The figure shows three views and two pictorial views of one solid part (mm, origin at its lowest corner). Answer the questions. A direction names the side the tool comes from. Coordinates: 2 decimals unless noted, no trailing zeros. Write each loop counter-clockwise with the first axis right and the second up, starting at its lowest first coordinate (ties: lowest second). Pieces come first, ordered by that corner, then holes. Notation, with made-up numbers: M 24.5,25 L 68.5,25 A20 cw 68.5,50 Z; hole C -3.5,86.25 d4. An arc over 180 degrees is marked long. Answer as CSV lines item,"result".
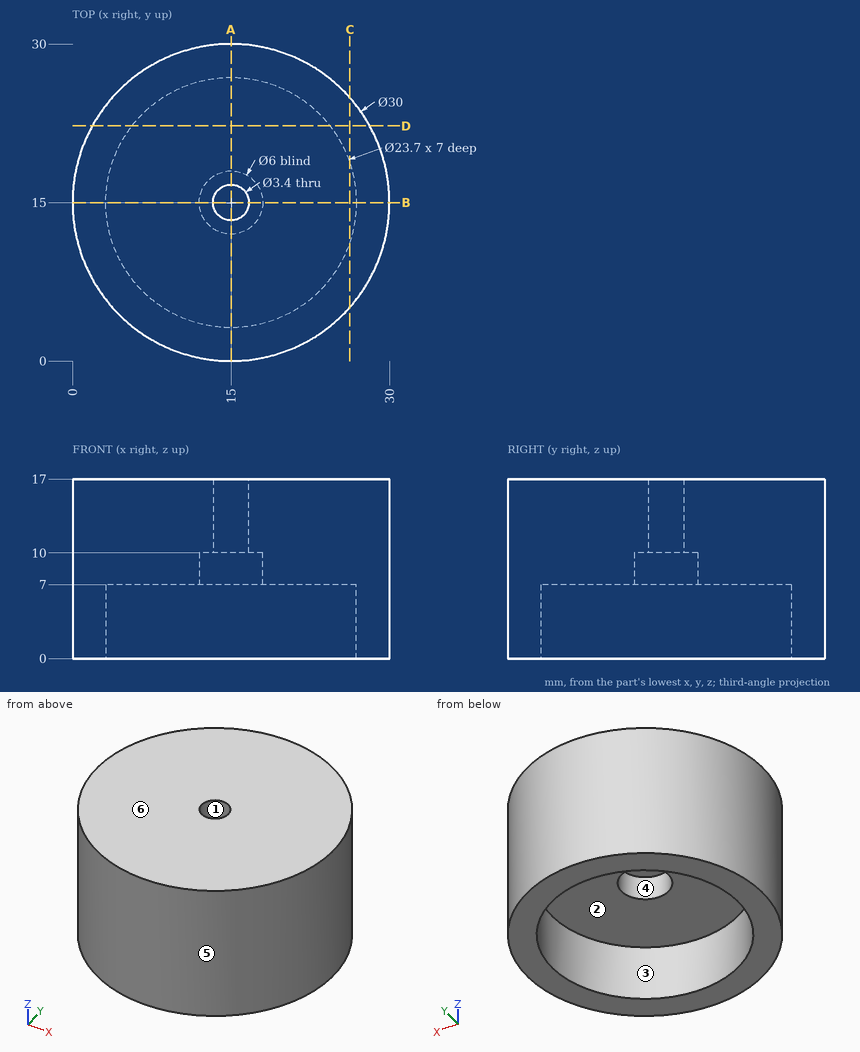
Q1. Flat-ended cylindrical pins translate along their axes: pin 1 Ø7 at (x, y) = (10.5, 20) entering from -Z; pin 2 Ø3 at (x, z) = (8.5, 11.5) entering from -Y; pin 3 Ø4 at (y, z) = (5.5, 6) entering from +X. Find the tip coordinate at first contact, or state that the pin passes through.
Output:
pin 1,"z = 7"
pin 2,"y = 0.86"
pin 3,"x = 27.99"
Q2. Find section D-D (y = 22.25). Give the vertices of the cut face in (x, z), and give its area (3 significant figures).
Output:
outline,"M 1.87,0 L 5.63,0 L 5.63,7 L 24.37,7 L 24.37,0 L 28.13,0 L 28.13,17 L 1.87,17 Z"
area,"315 mm2"
Q3. For the marked faces 1 and 2, determine the directions among +Z, -Z, +X, -X, +Y, -Y from which every point of the face is accessible in a straight line to the end or side of a thin tool.
Output:
face 1,"+Z, -Z"
face 2,"-Z"
Q4. Straight lines are drawn through the part: line 1 (Y direction, x = 15, z = 1.75); line 2 (Y direction, x = 15, z = 8.25); line 3 (Z direction, x = 12.75, y = 26.25). For each, find the intervals that lie inside material, in ascending order.
Output:
line 1,"0 to 3.15, 26.85 to 30"
line 2,"0 to 12, 18 to 30"
line 3,"7 to 17"
Q5. The mould has two halves that part along X. Classify the marked faces 3, 4, 5 and 6: pulls with the +X half, pulls with the -X half, needs draft (parallel to the pull), parting line crosses it, or undercut.
Output:
face 3,"undercut"
face 4,"undercut"
face 5,"parting line crosses it"
face 6,"needs draft"
Q6. Find section C-C (x = 26.25). Give the vertices of the cut face in (y, z).
Output:
outline,"M 5.08,0 L 11.28,0 L 11.28,7 L 18.72,7 L 18.72,0 L 24.92,0 L 24.92,17 L 5.08,17 Z"
Q7. Find section A-A (x = 15). Give the vertices of the cut face in (y, z), and give its area (3 significant figures).
Output:
outline,"M 0,0 L 3.15,0 L 3.15,7 L 12,7 L 12,10 L 13.3,10 L 13.3,17 L 0,17 Z; M 16.7,10 L 18,10 L 18,7 L 26.85,7 L 26.85,0 L 30,0 L 30,17 L 16.7,17 Z"
area,"302 mm2"
